Check sheet for the modelled part. Datum: model origin and axes. Units: mm. Face numbers are marked on the shaded views. A direction names the side the tool comes from. Give positions to 0.01 mm unless a question says otherwise; leave off trailing zeros. Order: outer loops, then holes, each group sorted by start corner. A loop starts at its lowest first (then second) coordinate and runs counter-clockwise, first axis right, second up.
```python
from build123d import *

# Parameters (mm, degrees)
BOSS_EXTRUDE1_DEPTH = 2
SKETCH4_W           = 4
SKETCH4_H           = 210
BOSS_EXTRUDE2_DEPTH = 2
CHAMFER1_SIZE       = 2


with BuildPart() as part:
    # Sketch3 → Boss-Extrude1 (new body)
    with BuildSketch(Plane.XY):
        Polygon((0, 50.432314919), (25, 50.432314919), (25, 250.584553029), (52.383760544, 279.950040998), (34.099918003, 297), (0, 260.432314919), align=None)
    extrude(amount=BOSS_EXTRUDE1_DEPTH)

    # Sketch4 → Boss-Extrude2 (add)
    with BuildSketch(Plane.ZY):
        with Locations((2, 155.432314919)):
            Rectangle(SKETCH4_W, SKETCH4_H)
    extrude(amount=BOSS_EXTRUDE2_DEPTH)

    # Chamfer1
    chamfer1_edges = [part.edges().sort_by_distance(p)[0] for p in [
        (38.691880272, 265.267297014, 0),
        (25, 150.508433974, 0),
    ]]
    chamfer(chamfer1_edges, length=CHAMFER1_SIZE - 0.0001)  # a hair under: the kernel refuses the full size


solid = part.part
```
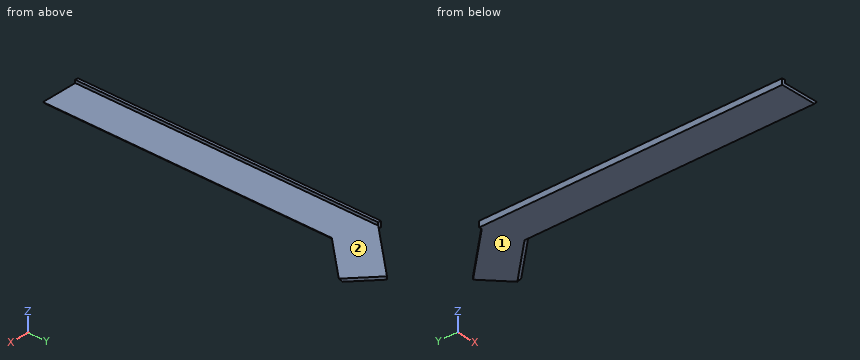
(1) Set-up check for the marked faces 1 and 2: record each of +Z, -Z, +X, -X, +Y, -Y from which the full face is reachable in a straight line by a thin tool's end or side.
Response values:
face 1: -Z, +X, -X, +Y, -Y
face 2: +Z, +X, +Y, -Y
(2) Gauge pin test, flat ends, axial feed: pin 1 Ø15.5 at (x, y) = (26.5, 227.5) entering from +Z; pin 2 Ø1.5 at (x, z) = (34.5, 2) entering from -Y; pin 3 Ø1.6 at (x, z) = (-1, 3) entering from +Y. Record the tip position at first contact, or that the pin passes through.
Response values:
pin 1: stops at z = 2
pin 2: stops at y = 259.97
pin 3: stops at y = 260.43
(3) Material ranges on L1, parallel to X at y = 174, z = 3.4; L2, parallel to Z at x = 12, y = 188.5; L3, parallel to X at y = 199.5, z = 1.95, recorded low to high.
Response values:
L1: x = -2 to 0
L2: z = 0 to 2
L3: x = -2 to 24.95
(4) Cross-section at B-B on z = 3.35. Enter the section's corners in (x, y).
Response values:
outline: (-2, 50.43) - (0, 50.43) - (0, 260.43) - (-2, 260.43) - close
